Read the model definition and answer for the solid it produces. Units are mm, in the model's axes. Face numbers are marked on the shaded views. A direction names the side the tool comes from. Coordinates: 2 decimals unless noted, no trailing zeros. Write each loop counter-clockwise with the first axis right and the second up, starting at its lowest first coordinate (ties: lowest second). Pieces come first, ordered by that corner, then holes.
(1) The part is cut by section D-D, the plane z = 80.5. Determine the outline of the cut face in (x, y), and give its area (3 significant figures).
(2) Straight lines are drawn through the part: line 1 along Y through (x, z) = (-299.55, 86); line 2 along Y through (x, z) = (-321.2, 86); line 3 along X through (y, z) = (50.5, 88). For each, find the intervals that lie inside material, in ascending order.
(3) The part is cut by section A-A, the plane y = 63. Determine the outline of the cut face in (x, z), and give its area (3 significant figures).
(4) Determine the mould class of the marked faces 6, 7 and 8 for opening direction Y: pulls with the +Y half, pulls with the -Y half, needs draft (parallel to the pull), parting line crosses it, or undercut.
(5) The part is cut by section C-C, the plane y = 69. Determine the outline of the cut face in (x, z), and give its area (3 significant figures).
(6) Which of the six approach directions +Z, -Z, +X, -X, +Y, -Y give full straight-line access (tool end or side, diameter ignored) to the marked faces 1, 2, 3, 4 and 5?
(7) The part is cut by section B-B, the plane x = -307.25. Determine the outline of the cut face in (y, z), and give its area (3 significant figures).
(8) Given pin 1 (2 mm diameter, centred on x = -306.5, z = 58.5, fed in from -Y); pin 2 (6 mm diameter, centred on x = -308, z = 87, fed in from +Y); pin 3 (7 mm diameter, centred on x = -308.5, y = 58.5, fed in from +Z); pin 4 (9.5 mm diameter, centred on y = 62, z = 86, fed in from +X), each flat-ended and moving along its own axis, determine where each tip first touches the part or whether it passes through.
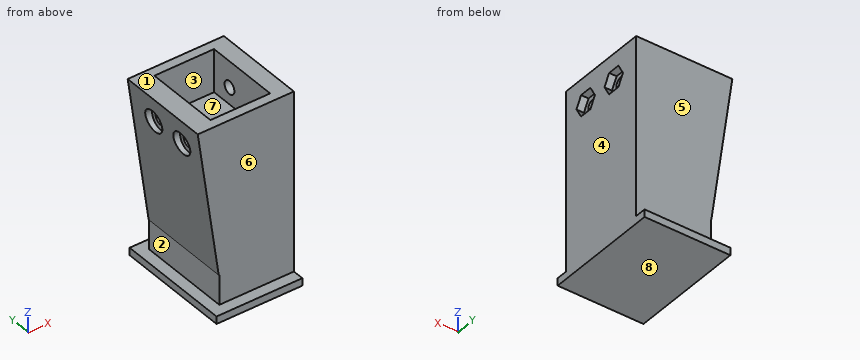
```python
from build123d import *

# Parameters (mm, degrees)
PRISM008_DEPTH            = 10
PRISM008_ROLL_ANGLE       = -90
CYLINDER111_R             = 3
CYLINDER111_DEPTH         = 32
CYLINDER111_ROLL_ANGLE    = -90
CYLINDER112_R             = 3
CYLINDER112_DEPTH         = 32
CYLINDER112_ROLL_ANGLE    = -90
BOX117_W                  = 20
BOX117_H                  = 16
BOX117_DEPTH              = 28
CYLINDER113_R             = 1.75
CYLINDER113_DEPTH         = 32
CYLINDER113_ROLL_ANGLE    = -90
CYLINDER114_R             = 1.75
CYLINDER114_DEPTH         = 32
CYLINDER114_ROLL_ANGLE    = -90
PRISM007_DEPTH            = 10
PRISM007_ROLL_ANGLE       = -90
FUSION079_ROLL_ANGLE      = 90
FUSION079_PLACEMENT_ANGLE = 180
BOX115_W                  = 2
BOX115_H                  = 23
BOX115_DEPTH              = 3
BOX110_W                  = 50
BOX110_H                  = 25
BOX110_DEPTH              = 20
BOX114_W                  = 2
BOX114_H                  = 25
BOX114_DEPTH              = 3
BOX113_W                  = 10
BOX113_H                  = 25
BOX113_DEPTH              = 10
BOX112_W                  = 30
BOX112_H                  = 30
BOX112_DEPTH              = 30
BOX112_PITCH_ANGLE        = 90
BOX111_W                  = 50
BOX111_H                  = 25
BOX111_DEPTH              = 6
BOX111_PITCH_ANGLE        = 8
FUSION077_PLACEMENT_ANGLE = -90
BOX116_W                  = 2
BOX116_H                  = 23
BOX116_DEPTH              = 3
CUT138_ROLL_ANGLE         = 90
CUT138_PLACEMENT_ANGLE    = -90


with BuildPart() as prisma008:
    # Prism008 → Prism008 (new body)
    with BuildSketch(Plane.XY):
        Polygon((3.3, 0), (1.65, 2.857884), (-1.65, 2.857884), (-3.3, 0), (-1.65, -2.857884), (1.65, -2.857884), align=None)
    extrude(amount=PRISM008_DEPTH)


with BuildPart() as prisma008_1:
    # Prism008 roll: moved
    add(prisma008.part.rotate(Axis((0, 0, 0), (1, 0, 0)), PRISM008_ROLL_ANGLE))


with BuildPart() as prisma008_2:
    # Prism008 placement: moved
    add(prisma008_1.part.moved(Location((8, 85, 84))))


with BuildPart() as cilindro038:
    # Cylinder111 → Cylinder111 (new body)
    with BuildSketch(Plane.XY):
        Circle(CYLINDER111_R)
    extrude(amount=CYLINDER111_DEPTH)


with BuildPart() as cilindro038_1:
    # Cylinder111 roll: moved
    add(cilindro038.part.rotate(Axis((0, 0, 0), (1, 0, 0)), CYLINDER111_ROLL_ANGLE))


with BuildPart() as cilindro038_2:
    # Cylinder111 placement: moved
    add(cilindro038_1.part.moved(Location((18, 116, 84))))


with BuildPart() as cilindro039:
    # Cylinder112 → Cylinder112 (new body)
    with BuildSketch(Plane.XY):
        Circle(CYLINDER112_R)
    extrude(amount=CYLINDER112_DEPTH)


with BuildPart() as cilindro039_1:
    # Cylinder112 roll: moved
    add(cilindro039.part.rotate(Axis((0, 0, 0), (1, 0, 0)), CYLINDER112_ROLL_ANGLE))


with BuildPart() as cilindro039_2:
    # Cylinder112 placement: moved
    add(cilindro039_1.part.moved(Location((8, 116, 84))))


with BuildPart() as cubo055:
    # Box117 → Box117 (new body)
    with BuildSketch(Plane(origin=(3.5, 97.5, 79.5), x_dir=(1, 0, 0), z_dir=(0, 0, 1))):
        with Locations((10, 8)):
            Rectangle(BOX117_W, BOX117_H)
    extrude(amount=BOX117_DEPTH)


with BuildPart() as cilindro040:
    # Cylinder113 → Cylinder113 (new body)
    with BuildSketch(Plane.XY):
        Circle(CYLINDER113_R)
    extrude(amount=CYLINDER113_DEPTH)


with BuildPart() as cilindro040_1:
    # Cylinder113 roll: moved
    add(cilindro040.part.rotate(Axis((0, 0, 0), (1, 0, 0)), CYLINDER113_ROLL_ANGLE))


with BuildPart() as cilindro040_2:
    # Cylinder113 placement: moved
    add(cilindro040_1.part.moved(Location((18, 90, 84))))


with BuildPart() as cilindro041:
    # Cylinder114 → Cylinder114 (new body)
    with BuildSketch(Plane.XY):
        Circle(CYLINDER114_R)
    extrude(amount=CYLINDER114_DEPTH)


with BuildPart() as cilindro041_1:
    # Cylinder114 roll: moved
    add(cilindro041.part.rotate(Axis((0, 0, 0), (1, 0, 0)), CYLINDER114_ROLL_ANGLE))


with BuildPart() as cilindro041_2:
    # Cylinder114 placement: moved
    add(cilindro041_1.part.moved(Location((8, 90, 84))))


with BuildPart() as arm_positive_cut003:
    # Prism007 → Prism007 (new body)
    with BuildSketch(Plane.XY):
        Polygon((3.3, 0), (1.65, 2.857884), (-1.65, 2.857884), (-3.3, 0), (-1.65, -2.857884), (1.65, -2.857884), align=None)
    extrude(amount=PRISM007_DEPTH)


with BuildPart() as arm_positive_cut003_1:
    # Prism007 roll: moved
    add(arm_positive_cut003.part.rotate(Axis((0, 0, 0), (1, 0, 0)), PRISM007_ROLL_ANGLE))


with BuildPart() as arm_positive_cut003_2:
    # Prism007 placement: moved
    add(arm_positive_cut003_1.part.moved(Location((18, 85, 84))))

    # Fusion079: union Prisma008, Cilindro038, Cilindro039, Cubo055, Cilindro040, Cilindro041
    add(prisma008_2.part)
    add(cilindro038_2.part)
    add(cilindro039_2.part)
    add(cubo055.part)
    add(cilindro040_2.part)
    add(cilindro041_2.part)


with BuildPart() as arm_positive_cut003_3:
    # Fusion079 roll: moved
    add(arm_positive_cut003_2.part.rotate(Axis((0, 0, 0), (1, 0, 0)), FUSION079_ROLL_ANGLE))


with BuildPart() as arm_positive_cut003_4:
    # Fusion079 placement: moved
    add(arm_positive_cut003_3.part.moved(Location((26, -91, -93))).rotate(Axis((26, -91, -93), (0, 0, 1)), FUSION079_PLACEMENT_ANGLE))


with BuildPart() as cubo053:
    # Box115 → Box115 (new body)
    with BuildSketch(Plane(origin=(0, -48, 0), x_dir=(0, -1, 0), z_dir=(-1, 0, 0))):
        with Locations((1, 11.5)):
            Rectangle(BOX115_W, BOX115_H)
    extrude(amount=BOX115_DEPTH)


with BuildPart() as cubo048:
    # Box110 → Box110 (new body)
    with BuildSketch(Plane.XY):
        with Locations((25, 12.5)):
            Rectangle(BOX110_W, BOX110_H)
    extrude(amount=BOX110_DEPTH)


with BuildPart() as cubo052:
    # Box114 → Box114 (new body)
    with BuildSketch(Plane(origin=(48, 0, 20), x_dir=(1, 0, 0), z_dir=(0, 0, 1))):
        with Locations((1, 12.5)):
            Rectangle(BOX114_W, BOX114_H)
    extrude(amount=BOX114_DEPTH)


with BuildPart() as cubo051:
    # Box113 → Box113 (new body)
    with BuildSketch(Plane(origin=(-10, 0, 16), x_dir=(1, 0, 0), z_dir=(0, 0, 1))):
        with Locations((5, 12.5)):
            Rectangle(BOX113_W, BOX113_H)
    extrude(amount=BOX113_DEPTH)


with BuildPart() as cubo050:
    # Box112 → Box112 (new body)
    with BuildSketch(Plane.XY):
        with Locations((15, 15)):
            Rectangle(BOX112_W, BOX112_H)
    extrude(amount=BOX112_DEPTH)


with BuildPart() as cubo050_1:
    # Box112 pitch: moved
    add(cubo050.part.rotate(Axis((0, 0, 0), (0, 1, 0)), BOX112_PITCH_ANGLE))


with BuildPart() as cubo050_2:
    # Box112 placement: moved
    add(cubo050_1.part.moved(Location((40, 0, 30))))


with BuildPart() as brazo002:
    # Box111 → Box111 (new body)
    with BuildSketch(Plane.XY):
        with Locations((25, 12.5)):
            Rectangle(BOX111_W, BOX111_H)
    extrude(amount=BOX111_DEPTH)


with BuildPart() as brazo002_1:
    # Box111 pitch: moved
    add(brazo002.part.rotate(Axis((0, 0, 0), (0, 1, 0)), BOX111_PITCH_ANGLE))


with BuildPart() as brazo002_2:
    # Box111 placement: moved
    add(brazo002_1.part.moved(Location((-2, 0, 20))))

    # Cut136: cut Cubo050
    add(cubo050_2.part, mode=Mode.SUBTRACT)

    # Cut137: cut Cubo051
    add(cubo051.part, mode=Mode.SUBTRACT)

    # Fusion077: union Cubo048, Cubo052
    add(cubo048.part)
    add(cubo052.part)


with BuildPart() as brazo002_3:
    # Fusion077 placement: moved
    add(brazo002_2.part.rotate(Axis((0, 0, 0), (0, 0, 1)), FUSION077_PLACEMENT_ANGLE))


with BuildPart() as cut138:
    # Box116 → Box116 (new body)
    with BuildSketch(Plane(origin=(28, -48, 0), x_dir=(0, -1, 0), z_dir=(-1, 0, 0))):
        with Locations((1, 11.5)):
            Rectangle(BOX116_W, BOX116_H)
    extrude(amount=BOX116_DEPTH)

    # Fusion078: union Cubo053, brazo002
    add(cubo053.part)
    add(brazo002_3.part)

    # Cut138: cut arm-positive-cut003
    add(arm_positive_cut003_4.part, mode=Mode.SUBTRACT)


with BuildPart() as cut138_1:
    # Cut138 roll: moved
    add(cut138.part.rotate(Axis((0, 0, 0), (1, 0, 0)), CUT138_ROLL_ANGLE))


with BuildPart() as cut138_2:
    # Cut138 placement: moved
    add(cut138_1.part.moved(Location((-297, 70, 93))).rotate(Axis((-297, 70, 93), (0, 0, 1)), CUT138_PLACEMENT_ANGLE))


solid = cut138_2.part
```
Computed:
1. outline: (-321.02, 45) - (-297, 45) - (-297, 70) - (-321.02, 70) - close
1. area: 601 mm2
2. line 1: y = 45 to 50.25, 53.75 to 60.25, 63.75 to 70
2. line 2: y = 45 to 49, 55 to 59, 65 to 70
2. line 3: x = -320 to -317.5, -301.5 to -299
3. outline: (-322.78, 93) - (-322.19, 88.83) - (-320, 88.83) - (-320, 87.44) - (-317.5, 87.44) - (-317.5, 93) - close; (-321.4, 83.17) - (-317.16, 53) - (-317, 53) - (-317, 45) - (-320, 45) - (-320, 43) - (-297, 43) - (-297, 83.14) - (-299, 83.14) - (-299, 84.56) - (-301.5, 84.56) - (-301.5, 81.5) - (-317.5, 81.5) - (-317.5, 84.56) - (-320, 84.56) - (-320, 83.17) - close; (-301.5, 87.44) - (-299, 87.44) - (-299, 88.86) - (-297, 88.86) - (-297, 93) - (-301.5, 93) - close
3. area: 905 mm2
4. face 6: pulls with the -Y half
4. face 7: undercut
4. face 8: needs draft
5. outline: (-322.78, 93) - (-317.16, 53) - (-317, 53) - (-317, 45) - (-320, 45) - (-320, 43) - (-297, 43) - (-297, 93) - close
5. area: 1,120 mm2
6. face 1: +Z, +X, -X, +Y, -Y
6. face 2: -X, +Y, -Y
6. face 3: +Z
6. face 4: +Z, -Z, +X, +Y, -Y
6. face 5: +Z, +X, -X, +Y
7. outline: (42, 43) - (73, 43) - (73, 45) - (70, 45) - (70, 93) - (67.5, 93) - (67.5, 81.5) - (47.5, 81.5) - (47.5, 93) - (45, 93) - (45, 45) - (42, 45) - close
7. area: 1,030 mm2
8. pin 1: stops at y = 45
8. pin 2: stops at y = 70
8. pin 3: stops at z = 81.5
8. pin 4: stops at x = -297
